Build history of the part. All positions in model axes, mm. A direction names the side the tool comes from. Give positions to 0.01 mm unless a question says otherwise; leave off trailing zeros. Write each loop counter-clockwise with the first axis right and the second up, starting at its lowest first coordinate (ties: lowest second). Pieces come first, ordered by that corner, then holes. Notation, with made-up numbers: M 5,40.5 L 40,40.5 A20 cw 40,44.5 Z; hole C -35,9 d3. An arc over 180 degrees is marked long. Return JSON: item names as keys, results as strings. Group by question number.
Q1. Tool access for faces 4 (the flat face through (48, -13, -64.219)), 5 (the flat face through (-11.022, -37.567, 52.659)), 6 (the flat face through (-9.263, -37.567, -52.181)), 7 (the flat face through (-30.53, -38, -3)): list every direction of +Z, -Z, +X, -X, +Y, -Y with a clear straight run to the whole face (end or side of a thin tool).
Q2. Band-saw the part on A-A, the plane z = -44.5. Give the cut face in (x, y), then the cut area to 3 significant figures.
Q3. Wall check: probe 1 along X at (y, z) = (-8, 39.5); probe 2 along X at (y, z) = (-15.5, -35); probe 3 along Z at (x, y) = (-62.5, -15.5). Give the ranges that are in metal, low to high.
Q4. Band-saw the part on D-D, the plane z = 10.5. Give the cut face in (x, y), then the cut area to 3 significant figures.
Q5. Band-saw the part on B-B, the plane x = 74. Give the cut face in (y, z).
Q6. Flat gauge pins, fed straight in: pin 1 Ø4 at (x, y) = (6.5, -49.5) entering from +Z; pin 2 Ø8.5 at (y, z) = (-19, -5.5) entering from -X; pin 3 Ø10 at (y, z) = (-55.5, 50.5) entering from +X. Where does each tip first touch, or does it go through?
Q7. Band-saw the part on C-C, the plane y = -33. Give the cut face in (x, z), then the cut area to 3 significant figures.
Q8. Pull direction Z, two halves, no side cores. Call faces 1 (the flat face through (52, -38, -72.941)), 2 (the flat face through (1, -13, 16.393)), 3 (the flat face through (0, -38, 27.522)): +Z half, -Z half, draft (parallel to the pull), parting line (faces both ways), or undercut.
from build123d import *

# Parameters (mm, degrees)
F2_DEPTH = 76.2
F3_DEPTH = 25.4


with BuildPart() as f2:
    # F0 (on Front) → F2 (new body)
    with BuildSketch(Plane.XZ):
        Polygon((-18.799344, 72.941445), (-76.851711, 72.941445), (-44.065658, 0), (-30.53013, 0), (-30.53013, -5.263816), (-42.862501, -5.263816), (-79.258025, -72.941445), (-15.490658, -72.941445), (-2.857502, -30.83092), (-2.857502, -23.311185), (5.263818, -23.311185), (5.263818, -29.326973), (26.319075, -72.941445), (78.65645, -72.941445), (40.756974, -6.767763), (33.538029, -6.767763), (33.538029, -2.8575), (41.358553, -2.8575), (87.379344, 72.941445), (22.408813, 72.941445), (3.759871, 32.334868), (3.759871, 27.522238), (-3.459081, 27.522238), (-3.459081, 32.93645), align=None)
    extrude(amount=F2_DEPTH)

    # F1 (on Front) → F3 (cut)
    with BuildSketch(Plane.XZ):
        Polygon((-25.115922, 63.316189), (-59.105132, 63.316189), (-26.619868, 3.459079), (-26.619868, -8.271711), (-62.714607, -67.226447), (-20.30329, -67.226447), (-3.75987, -19.70171), (7.068554, -19.70171), (34.741186, -64.218551), (61.210655, -64.218551), (27.221451, -7.670132), (27.221451, 0), (64.519338, 60.909871), (32.635659, 60.909871), (6.466975, 16.393026), (-3.75987, 16.393026), align=None)
    extrude(amount=F3_DEPTH, mode=Mode.SUBTRACT)


solid = f2.part
From the geometry:
{
 "1": {"face 4": "+Y", "face 5": "+Z, +Y, -Y", "face 6": "-Z, +Y, -Y", "face 7": "-X, +Y, -Y"},
 "2": {"outline": "M -63.96,-76.2 L -6.96,-76.2 L -6.96,0 L -12.39,0 L -12.39,-25.4 L -48.8,-25.4 L -48.8,0 L -63.96,0 Z; M 12.59,-76.2 L 62.37,-76.2 L 62.37,0 L 49.36,0 L 49.36,-25.4 L 22.48,-25.4 L 22.48,0 L 12.59,0 Z", "area": "6,530 mm^2"},
 "3": {"probe 1": "x = -61.82 to -46.18, -14.28 to -5.98, 7.05 to 20.05, 51.41 to 67.08", "probe 2": "x = -58.85 to -42.98, -9.09 to -4.11, 8 to 16.58, 43.65 to 56.93", "probe 3": "z = -72.94 to -67.23, -66.88 to -41.78, 41.01 to 72.94"},
 "4": {"outline": "M -48.79,-76.2 L 49.47,-76.2 L 49.47,0 L 33.65,0 L 33.65,-25.4 L -30.44,-25.4 L -30.44,0 L -48.79,0 Z", "area": "5,860 mm^2"},
 "5": {"outline": "M -76.2,-72.94 L 0,-72.94 L 0,-64.81 L -76.2,-64.81 Z; M -76.2,50.9 L 0,50.9 L 0,72.94 L -76.2,72.94 Z"},
 "6": {"pin 1": "stops at z = 42.66", "pin 2": "stops at x = -45.28", "pin 3": "stops at x = 76.79"},
 "7": {"outline": "M -79.26,-72.94 L -15.49,-72.94 L -2.86,-30.83 L -2.86,-23.31 L 5.26,-23.31 L 5.26,-29.33 L 26.32,-72.94 L 78.66,-72.94 L 40.76,-6.77 L 33.54,-6.77 L 33.54,-2.86 L 41.36,-2.86 L 87.38,72.94 L 22.41,72.94 L 3.76,32.33 L 3.76,27.52 L -3.46,27.52 L -3.46,32.94 L -18.8,72.94 L -76.85,72.94 L -44.07,0 L -30.53,0 L -30.53,-5.26 L -42.86,-5.26 Z", "area": "15,500 mm^2"},
 "8": {"face 1": "-Z half", "face 2": "undercut", "face 3": "+Z half"}
}
